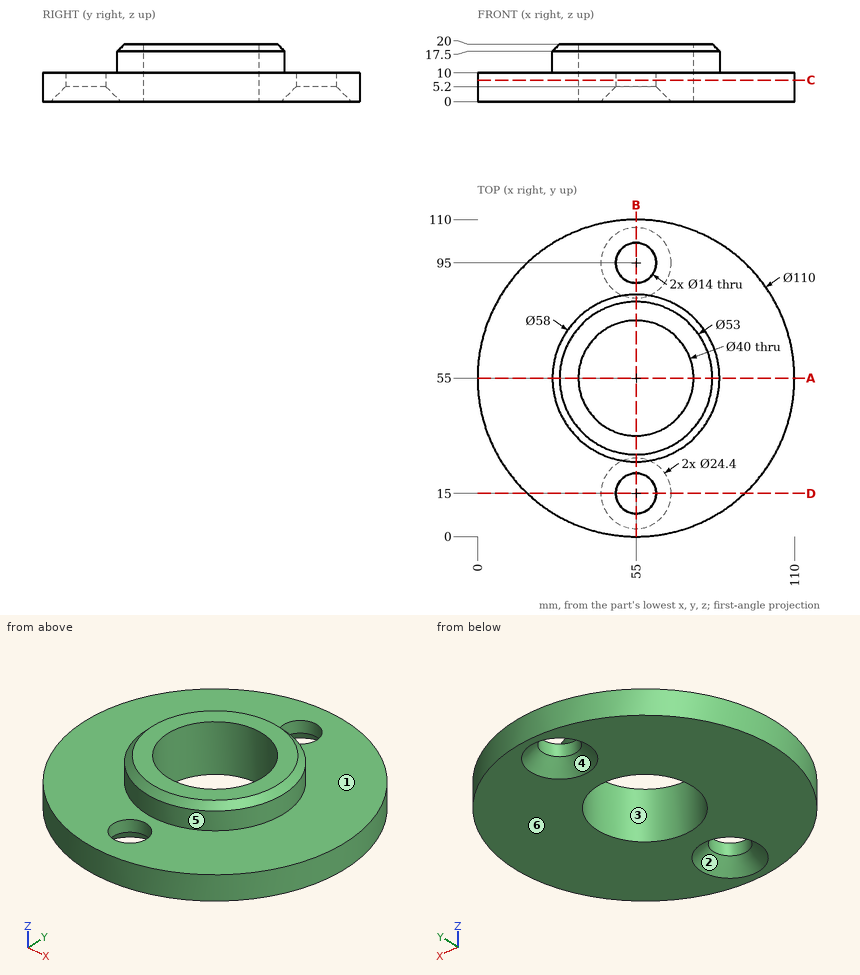
Geometry: see drawing. Coordinates: mm, zero at the bounding-box minimum. A direction names the side the tool comes from. Give positions to 0.01 mm unless a question says otherwise; leave off trailing zeros. Order: outer loops, then holes, each group sorted by start corner. A loop starts at its lowest first (then second) coordinate and runs counter-clockwise, first axis right, second up. Notation, with made-up numbers: (-25, 46) - (32, 46) arc R17 ccw to (32, 52) - close; hole circle Ø5 at (54, 69). An arc over 180 degrees is marked (long way). Use a Markdown table: item, result.
(1) Access query for the marked faces 1 and 2. Directions: +Z, -Z, +X, -X, +Y, -Y. A direction counts if a zero-diameter tool reaches every point of the face in a straight line with its end or side. Return the directions, or none.
Computed values:
| item | result |
|---|---|
| face 1 | +Z |
| face 2 | -Z |
(2) Section query C-C (z = 7.5). Output: boundary loops of the cut face in (x, y), then the cut area to 3 significant figures.
Computed values:
| item | result |
|---|---|
| outline | circle Ø110 at (55, 55); hole circle Ø40 at (55, 55); hole circle Ø14 at (55, 15); hole circle Ø14 at (55, 95) |
| area | 7,940 mm2 |
(3) Draft query along X for the marked faces 3, 4, 5 and 6. Return one class per face: released by +X, released by -X, zero draft, split by the parting line, or undercut.
Computed values:
| item | result |
|---|---|
| face 3 | undercut |
| face 4 | undercut |
| face 5 | split by the parting line |
| face 6 | zero draft |
(4) Pin query (flat end, axial travel): pin 1 (5 mm diameter, centred on x = 18, y = 72, fed in from +Z); pin 2 (1 mm diameter, centred on x = 26.5, z = 8, fed in from +Y); pin 3 (22.5 mm diameter, centred on x = 55, y = 95, fed in from +Z). Return the tip coordinate at first contact, or that it passes through.
Computed values:
| item | result |
|---|---|
| pin 1 | stops at z = 10 |
| pin 2 | stops at y = 102.34 |
| pin 3 | stops at z = 17.75 |
(5) Section query A-A (y = 55). Output: boundary loops of the cut face in (x, z), then the cut area to 3 significant figures.
Computed values:
| item | result |
|---|---|
| outline | (0, 0) - (35, 0) - (35, 20) - (28.5, 20) - (26, 17.5) - (26, 10) - (0, 10) - close; (75, 0) - (110, 0) - (110, 10) - (84, 10) - (84, 17.5) - (81.5, 20) - (75, 20) - close |
| area | 874 mm2 |
(6) Section query B-B (x = 55). Output: boundary loops of the cut face in (y, z).
Computed values:
| item | result |
|---|---|
| outline | (0, 0) - (2.8, 0) - (8, 5.2) - (8, 10) - (0, 10) - close; (22, 5.2) - (27.2, 0) - (35, 0) - (35, 20) - (28.5, 20) - (26, 17.5) - (26, 10) - (22, 10) - close; (75, 0) - (82.8, 0) - (88, 5.2) - (88, 10) - (84, 10) - (84, 17.5) - (81.5, 20) - (75, 20) - close; (102, 5.2) - (107.2, 0) - (110, 0) - (110, 10) - (102, 10) - close |
(7) Line query: line 1 (Y direction, x = 55, z = 8.4); line 2 (Y direction, x = 51, z = 9.25); line 3 (X direction, y = 15, z = 6.95). Output: solid intervals per line, ascending. Write a range as from..to.
Computed values:
| item | result |
|---|---|
| line 1 | y = 0..8, 22..35, 75..88, 102..110 |
| line 2 | y = 0.15..9.26, 20.74..35.4, 74.6..89.26, 100.74..109.85 |
| line 3 | x = 17.25..48, 62..92.75 |
(8) Section query D-D (y = 15). Output: boundary loops of the cut face in (x, z), then the cut area to 3 significant figures.
Computed values:
| item | result |
|---|---|
| outline | (17.25, 0) - (42.8, 0) - (48, 5.2) - (48, 10) - (17.25, 10) - close; (62, 5.2) - (67.2, 0) - (92.75, 0) - (92.75, 10) - (62, 10) - close |
| area | 588 mm2 |
